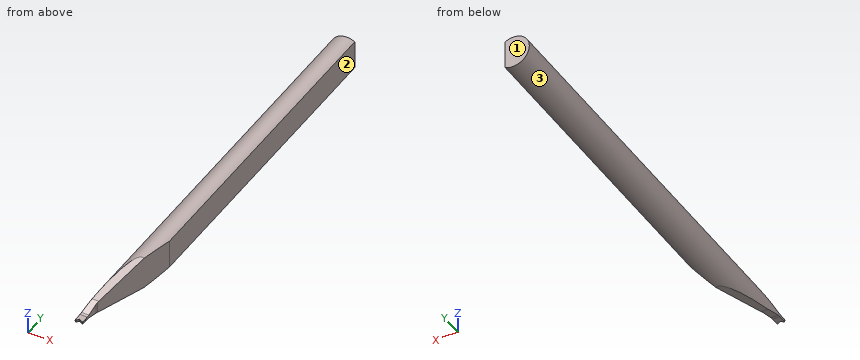
```python
from build123d import *

# Parameters (mm, degrees)
TD_REV_FEATURE_DEPTH            = 21.0312
ISA_REV_FEATURE_DEPTH           = 22.061040395
ISA_REV_FEATURE_DEPTH_BACK      = 22.061040395
BA_REV_FEATURE_DEPTH            = 22.061040395
BA_REV_FEATURE_DEPTH_BACK       = 22.061040395
SLB_REV_FEATURE_DEPTH           = 22.061040395
SLB_REV_FEATURE_DEPTH_BACK      = 22.061040395
VR_REV_FEATURE_DEPTH            = 22.061040395
VR_REV_FEATURE_DEPTH_BACK       = 22.061040395
ND_REV_FEATURE_DEPTH            = 22.061040503
ND_REV_FEATURE_DEPTH_BACK       = 22.061040503
REV_HOLE_CUT_FEATURE_DEPTH      = 22.162851782
REV_HOLE_CUT_FEATURE_DEPTH_BACK = 22.162851782
REV_F_FR_FEATURE_R              = 0.0254
REV_F_BR_FEATURE_R              = 0.0254


with BuildPart() as part:
    # td_rev_sketch → td_rev_feature (new body)
    with BuildSketch(Plane(origin=(0, 0, 0), x_dir=(1, 0, 0), z_dir=(0, 1, 0))):
        with BuildLine():
            Line((0.37592, -0.697645113), (0.37592, 0.697645113))
            ThreePointArc((0.37592, 0.697645113), (-0.79248, 0), (0.37592, -0.697645113))
        make_face()
    extrude(amount=TD_REV_FEATURE_DEPTH)

    # isa_rev_sketch → isa_rev_feature (cut, two sides: drawn at the far end of the back side and taken through both)
    with BuildSketch(Plane(origin=(0, 0, 0), x_dir=(0, 0, -1), z_dir=(1, 0, 0)).offset(-ISA_REV_FEATURE_DEPTH_BACK)):
        Polygon((8.398066277, 47.339699483), (0.79248, 4.2062763), (0.0508, 0), (-0.0508, 0), (-0.79248, 4.2062763), (-8.398066277, 47.339699483), (-8.398066277, -40.25795204), (8.398066277, -40.25795204), align=None)
    extrude(amount=ISA_REV_FEATURE_DEPTH + ISA_REV_FEATURE_DEPTH_BACK, mode=Mode.SUBTRACT)

    # ba_rev_sketch → ba_rev_feature (cut, two sides: drawn at the far end of the back side and taken through both)
    with BuildSketch(Plane.XY.offset(-BA_REV_FEATURE_DEPTH_BACK)):
        Polygon((-52.01559187, -9.04993148), (-0.69088, 0), (-0.428729423, 0.04622422), (0.37592, 4.609617863), (9.42585148, 55.934329733), (85.165346017, -15.675992153), (23.723902667, -80.660253365), align=None)
    extrude(amount=BA_REV_FEATURE_DEPTH + BA_REV_FEATURE_DEPTH_BACK, mode=Mode.SUBTRACT)

    # slb_rev_sketch → slb_rev_feature (cut, two sides: drawn at the far end of the back side and taken through both)
    with BuildSketch(Plane.XY.offset(-SLB_REV_FEATURE_DEPTH_BACK)):
        with BuildLine():
            Line((-0.43688, -52.09380084), (-0.43688, 0))
            Line((-0.43688, 0), (-0.43688, 1.143))
            ThreePointArc((-0.43688, 1.143), (-0.434946907, 1.187275117), (-0.429162339, 1.231213274))
            Line((-0.429162339, 1.231213274), (0.37592, 5.797062104))
            Line((0.37592, 5.797062104), (9.421913584, 57.099441055))
            Line((9.421913584, 57.099441055), (113.187433376, 47.730703366))
            Line((113.187433376, 47.730703366), (103.328639792, -61.462538529))
            Line((103.328639792, -61.462538529), (-0.43688, -52.09380084))
        make_face()
    extrude(amount=SLB_REV_FEATURE_DEPTH + SLB_REV_FEATURE_DEPTH_BACK, mode=Mode.SUBTRACT)

    # vr_rev_sketch → vr_rev_feature (cut, two sides: drawn at the far end of the back side and taken through both)
    with BuildSketch(Plane(origin=(0, 0, 0), x_dir=(0, 0, -1), z_dir=(1, 0, 0)).offset(-VR_REV_FEATURE_DEPTH_BACK)):
        with BuildLine():
            Line((12.638111697, 47.42606773), (0.79248, 3.217568389))
            Line((0.79248, 3.217568389), (0.07445968, 0.537880075))
            ThreePointArc((0.07445968, 0.537880075), (0.06149601, 0.472707306), (0.05715, 0.4064))
            Line((0.05715, 0.4064), (0.05715, 0))
            Line((0.05715, 0), (-0.05715, 0))
            Line((-0.05715, 0), (-0.05715, 0.4064))
            ThreePointArc((-0.05715, 0.4064), (-0.06149601, 0.472707306), (-0.07445968, 0.537880075))
            Line((-0.07445968, 0.537880075), (-0.79248, 3.217568389))
            Line((-0.79248, 3.217568389), (-12.638111697, 47.42606773))
            Line((-12.638111697, 47.42606773), (-12.638111697, -44.109944949))
            Line((-12.638111697, -44.109944949), (12.638111697, -44.109944949))
            Line((12.638111697, -44.109944949), (12.638111697, 47.42606773))
        make_face()
    extrude(amount=VR_REV_FEATURE_DEPTH + VR_REV_FEATURE_DEPTH_BACK, mode=Mode.SUBTRACT)

    # erw_rev_sketch → nd_rev_feature (cut, two sides: drawn at the far end of the back side and taken through both)
    with BuildSketch(Plane.XY.offset(-ND_REV_FEATURE_DEPTH_BACK)):
        with BuildLine():
            Line((-0.73406, 0), (-0.668068864, 0.1143))
            ThreePointArc((-0.668068864, 0.1143), (-0.652645823, 0.126134516), (-0.633371819, 0.123597045))
            Line((-0.633371819, 0.123597045), (-0.476954112, 0.03328924))
            Line((-0.476954112, 0.03328924), (-0.419295457, 0))
            Line((-0.419295457, 0), (-0.73406, 0))
        make_face()
    extrude(amount=ND_REV_FEATURE_DEPTH + ND_REV_FEATURE_DEPTH_BACK, mode=Mode.SUBTRACT)


with BuildPart() as body_2:
    # rev_hole_sketch → rev_hole_feature (revolve)
    with BuildSketch(Plane.XY):
        Polygon((-0.703570884, -0.035921024), (-0.721531396, -0.017960512), (1.354405484, 2.057976368), (2.104599043, 1.307782809), (-0.395400957, 0.272248903), align=None)
    revolve(axis=Axis((-0.721531396, -0.017960512, 0), (0.7071067811865462, 0.7071067811865489, 0)))

    # rev_hole_cut_sketch → rev_hole_cut_feature (cut, two sides: drawn at the far end of the back side and taken through both)
    with BuildSketch(Plane.XY.offset(-REV_HOLE_CUT_FEATURE_DEPTH_BACK)):
        Polygon((-46.14120993, 26.397559629), (-0.79248, 0.215458196), (-0.419295457, 0), (44.929434473, -26.182101432), (-7.434768392, -116.879561292), (-98.505412795, -64.299900231), align=None)
    extrude(amount=REV_HOLE_CUT_FEATURE_DEPTH + REV_HOLE_CUT_FEATURE_DEPTH_BACK, mode=Mode.SUBTRACT)


with BuildPart() as part_1:
    add(part.part)

    # rev_hole_combine: cut body 2
    add(body_2.part, mode=Mode.SUBTRACT)

    # rev_f_fr_feature
    rev_f_fr_feature_edges = [part_1.edges().sort_by_distance(p)[0] for p in [
        (-0.79248, 0, 0),
    ]]
    fillet(rev_f_fr_feature_edges, radius=REV_F_FR_FEATURE_R)

    # rev_f_br_feature
    rev_f_br_feature_edges = [part_1.edges().sort_by_distance(p)[0] for p in [
        (-0.73406, 0, 0),
    ]]
    fillet(rev_f_br_feature_edges, radius=REV_F_BR_FEATURE_R)


solid = part_1.part
```
Part model, mm, in its own coordinate system. Face numbers are marked on the shaded views. Give positions to 0.01 mm unless a question says otherwise; leave off trailing zeros. Order: outer loops, then holes, each group sorted by start corner. A loop starts at its lowest first (then second) coordinate and runs counter-clockwise, first axis right, second up. Notation, with made-up numbers: (43.25, 21.25) - (75.25, 21.25) arc R23 ccw to (75.25, 44.25) - close; hole circle Ø8 at (86, -4.75). An arc over 180 degrees is marked (long way). Use one line per item in the form item = value.
Item 1: Slice it at B-B on y = 2. Give the cut face in (x, z), and give its area (3 significant figures).
Solution:
outline = (-0.68, -0.4) - (-0.29, -0.4) - (-0.29, 0.4) - (-0.68, 0.4) arc R0.79 ccw to start
area = 0.374 mm2
Item 2: Slice it at A-A on y = 17.25. Give the cut face in (x, z).
Solution:
outline = (0.38, -0.7) - (0.38, 0.7) arc R0.79 ccw (long way) to start
Item 3: Two-plate mould, pull along X, no slides. Class the marked faces 1, 2 and 3: released by +X, released by -X, zero draft, split by the parting line, or undercut.
Solution:
face_1 = zero draft
face_2 = released by +X
face_3 = split by the parting line
Item 4: Probe probe 1 along X at (y, z) = (19.25, 0.2); probe 2 along Z at (x, y) = (0.1, 16); probe 3 along X at (y, z) = (18.25, 0.65). List the from-to ranges inside material, lowest first. Write a range as from..to.
Solution:
probe_1 = -0.77..0.38
probe_2 = -0.79..0.79
probe_3 = -0.45..0.38
